Could you check a few things on this drawing? It's one solid part, dimensions in mm from its lowest x, y, z. Give positions to 0.01 mm unless a question says otherwise; leave off trailing zeros. Loops run counter-clockwise (first coordinate to the right, second up) from the corner with the lowest first, then second, coordinate; pieces in that order, holes last. Notation, with made-up numbers: M 67.25,-12.5 L 81.25,-12.5 A19 ccw 81.25,11.5 Z; hole C 23,62.5 d11. An arc over 180 degrees is marked long. Answer in a Markdown table with one row per item. Add a question column.
1. If we section it at C-C on z = 3.5: Count the separate pieces of the cut face and the enclosed holes in it, then the cut area to 3 significant figures.
2. If we section it at D-D on x = 31.75: List the corners of the cut face in (y, z) for me (1 decimal).
3. If we section it at B-B on y = 12.7: List the corners of the cut face in (x, z) for me (3 decimals).
4. If we section it at A-A on y = 88.9: List the corners of the cut face in (x, z) for me (1 decimal), then the cut area to 3 significant figures.
5. I need wall thicknesses on line 1 along X through (y, z) = (13, 8); line 2 along Y through (x, z) = (10, 6.5) (3 decimals); line 3 along Y through (x, z) = (8, 8). Which ranges of each line are inside material? Lowest first, please. Write a range as from..to.
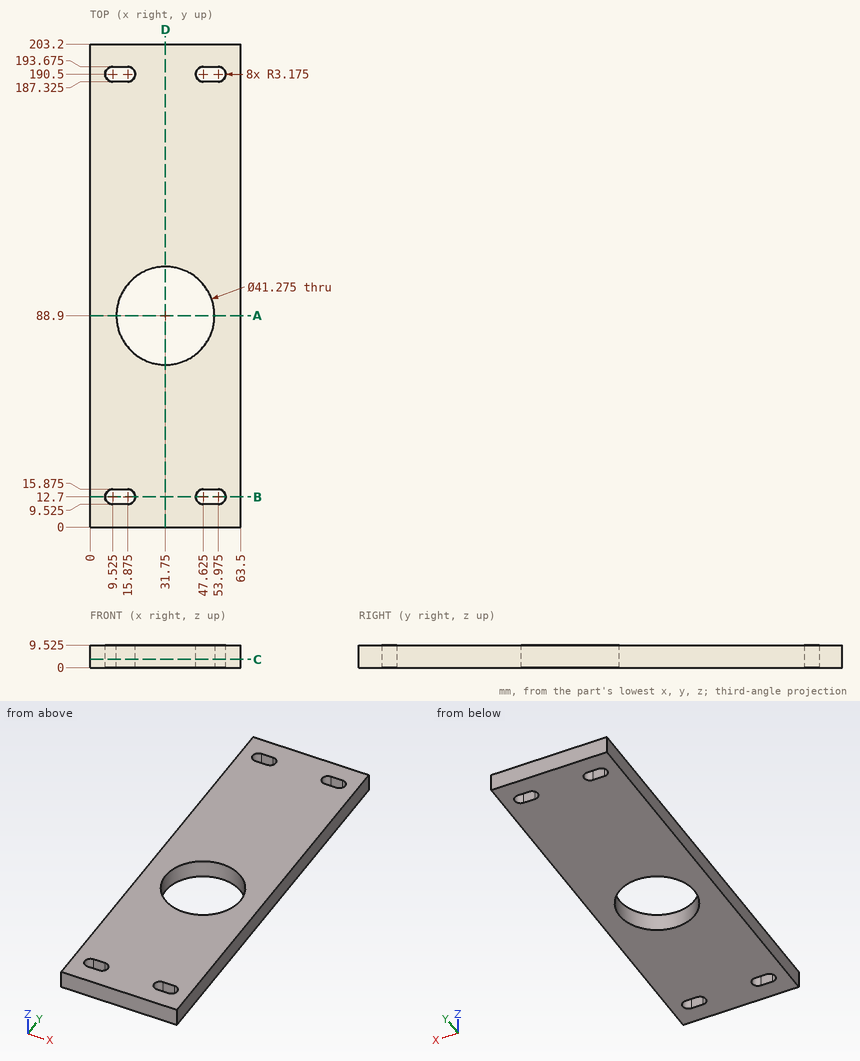
Results:
| question | item | result |
|---|---|---|
| 1 | separate pieces | 1 |
| 1 | enclosed holes | 5 |
| 1 | area | 11,300 mm2 |
| 2 | outline | M 0,0 L 68.3,0 L 68.3,9.5 L 0,9.5 Z; M 109.5,0 L 203.2,0 L 203.2,9.5 L 109.5,9.5 Z |
| 3 | outline | M 0,0 L 6.35,0 L 6.35,9.525 L 0,9.525 Z; M 19.05,0 L 44.45,0 L 44.45,9.525 L 19.05,9.525 Z; M 57.15,0 L 63.5,0 L 63.5,9.525 L 57.15,9.525 Z |
| 4 | outline | M 0,0 L 11.1,0 L 11.1,9.5 L 0,9.5 Z; M 52.4,0 L 63.5,0 L 63.5,9.5 L 52.4,9.5 Z |
| 4 | area | 212 mm2 |
| 5 | line 1 | 0..6.36, 19.04..44.46, 57.14..63.5 |
| 5 | line 2 | 0..9.525, 15.875..187.325, 193.675..203.2 |
| 5 | line 3 | 0..9.92, 15.48..187.72, 193.28..203.2 |
